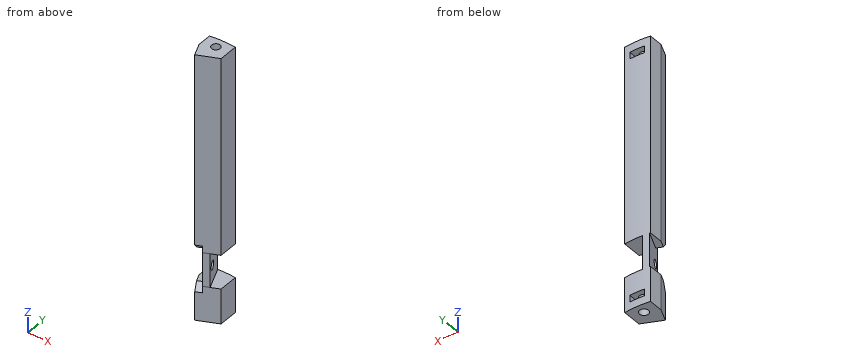
from build123d import *

# Parameters (mm, degrees)
BOSS_EXTRU_2_DEPTH       = 102.5
ESQUISSE8_R              = 1.75
ENL_V_MAT_EXTRU_5_DEPTH  = 11.5
ENL_V_START              = -3
ENL_V_MAT_EXTRU_6_DEPTH  = 2.6
ENL_V_START_2            = -89
ENL_V_MAT_EXTRU_11_DEPTH = 13
ESQUISSE15_R             = 1.625
ENL_V_MAT_EXTRU_12_DEPTH = 109.858621468
CHANFREIN1_SIZE          = 2.5
ESQUISSE16_R             = 1.65
ENL_V_MAT_EXTRU_13_DEPTH = 11.5
ENL_V_START_3            = -5.6
ENL_V_MAT_EXTRU_14_DEPTH = 2.6


with BuildPart() as part:
    # Esquisse3 → Boss.-Extru.2 (new body)
    with BuildSketch(Plane.XY):
        with BuildLine():
            Line((5, 29.665669478), (-2.833530831, 26.427314208))
            Line((-2.833530831, 26.427314208), (-5, 31.657633458))
            Line((-5, 31.657633458), (-5, 37.165171868))
            ThreePointArc((-5, 37.165171868), (0, 37.5), (5, 37.165171868))
            Line((5, 37.165171868), (5, 29.665669478))
        make_face()
    extrude(amount=BOSS_EXTRU_2_DEPTH)

    # Esquisse8 → Enlèv. mat.-Extru.5 (cut)
    with BuildSketch(Plane(origin=(0, 0, 0), x_dir=(-1, 0, 0), z_dir=(0, 0, -1))):
        with Locations((0, 33.75)):
            Circle(ESQUISSE8_R)
    extrude(amount=-ENL_V_MAT_EXTRU_5_DEPTH, mode=Mode.SUBTRACT)

    # Esquisse9 → Enlèv. mat.-Extru.6 (cut)
    with BuildSketch(Plane(origin=(0, 0, 0), x_dir=(-1, 0, 0), z_dir=(0, 0, -1)).offset(ENL_V_START)):
        with BuildLine():
            Line((-2.85, 37.391543162), (-2.85, 31.995448267))
            Line((-2.85, 31.995448267), (0, 30.35))
            Line((0, 30.35), (2.85, 31.995448267))
            Line((2.85, 31.995448267), (2.85, 37.391543162))
            ThreePointArc((2.85, 37.391543162), (0, 37.5), (-2.85, 37.391543162))
        make_face()
    extrude(amount=-ENL_V_MAT_EXTRU_6_DEPTH, mode=Mode.SUBTRACT)

    # Esquisse14 → Enlèv. mat.-Extru.11 (cut)
    with BuildSketch(Plane.XY.offset(102.5).offset(ENL_V_START_2)):
        with BuildLine():
            Line((-2.833530831, 26.427314208), (-0.564385746, 27.365371146))
            Line((-0.564385746, 27.365371146), (-4.642779542, 37.211484761))
            ThreePointArc((-4.642779542, 37.211484761), (-4.821445379, 37.188757232), (-5, 37.165171868))
            Line((-5, 37.165171868), (-5, 31.657633458))
            Line((-5, 31.657633458), (-2.833530831, 26.427314208))
        make_face()
        with BuildLine():
            Line((1.745788964, 28.320930853), (-0.564385746, 27.365371146))
            Line((-0.564385746, 27.365371146), (5, 29.665669478))
            Line((5, 29.665669478), (5, 37.165171868))
            ThreePointArc((5, 37.165171868), (1.48984988, 37.470392943), (-2.03345257, 37.444827021))
            Line((-2.03345257, 37.444827021), (1.745788964, 28.320930853))
        make_face()
    extrude(amount=ENL_V_MAT_EXTRU_11_DEPTH, mode=Mode.SUBTRACT)

    # Esquisse15 → Enlèv. mat.-Extru.12 (cut, through all)
    with BuildSketch(Plane(origin=(11.503085218, 4.764733906, 0), x_dir=(0, 0, -1), z_dir=(0.9238795325112864, 0.38268343236509095, 0))):
        with Locations(Location((-20, 28.49654364, 0), (0, 0, 90))):
            Circle(ESQUISSE15_R)
    extrude(amount=-ENL_V_MAT_EXTRU_12_DEPTH, mode=Mode.SUBTRACT)

    # Chanfrein1
    # the kernel refuses this chamfer: 2.5 mm, written as the material it takes off along each edge
    with BuildSketch(Plane(origin=(-8.775058658, 23.971106609, 13.5), x_dir=(0.010504495520027614, -0.025410210633805018, -0.9996219169112968), z_dir=(0.924146227220892, 0.38203893873974615, 0))) as chanfrein1_piece_1_section:
        Polygon((CHANFREIN1_SIZE * 0.999621916911, CHANFREIN1_SIZE * 0.0274958766106), (-CHANFREIN1_SIZE * 0.0274958766106, CHANFREIN1_SIZE * 0.999621916911), (0, 0), align=None)
    chanfrein1_piece_1 = extrude(amount=8.884603616, mode=Mode.PRIVATE)
    chanfrein1_piece_1 = split(chanfrein1_piece_1, bisect_by=Plane(origin=(-0.88361638, 28.136062073, 12.666666667), z_dir=(-0.9238795325112863, -0.382683432365091, 0)), keep=Keep.TOP, mode=Mode.PRIVATE)
    add(chanfrein1_piece_1, mode=Mode.SUBTRACT)
    with BuildSketch(Plane(origin=(-8.775058658, 23.971106609, 26.5), x_dir=(-0.38189449627778244, 0.9237968231608907, -0.027495876610586317), z_dir=(0.924146227220892, 0.38203893873974615, 0))) as chanfrein1_piece_2_section:
        Polygon((CHANFREIN1_SIZE * 0.999621916911, CHANFREIN1_SIZE * 0.0274958766106), (-CHANFREIN1_SIZE * 0.0274958766106, CHANFREIN1_SIZE * 0.999621916911), (0, 0), align=None)
    chanfrein1_piece_2 = extrude(amount=8.884603616, mode=Mode.PRIVATE)
    chanfrein1_piece_2 = split(chanfrein1_piece_2, bisect_by=Plane(origin=(-0.88361638, 28.136062073, 27.333333333), z_dir=(-0.9238795325112863, -0.382683432365091, 0)), keep=Keep.TOP, mode=Mode.PRIVATE)
    add(chanfrein1_piece_2, mode=Mode.SUBTRACT)

    # Esquisse16 → Enlèv. mat.-Extru.13 (cut)
    with BuildSketch(Plane.XY.offset(102.5)):
        with Locations((0, 33.75)):
            Circle(ESQUISSE16_R)
    extrude(amount=-ENL_V_MAT_EXTRU_13_DEPTH, mode=Mode.SUBTRACT)

    # Esquisse17 → Enlèv. mat.-Extru.14 (cut)
    with BuildSketch(Plane.XY.offset(102.5).offset(ENL_V_START_3)):
        with BuildLine():
            Line((-2.85, 37.391543162), (-2.85, 31.995448267))
            Line((-2.85, 31.995448267), (0, 30.35))
            Line((0, 30.35), (2.85, 31.995448267))
            Line((2.85, 31.995448267), (2.85, 37.391543162))
            ThreePointArc((2.85, 37.391543162), (0, 37.5), (-2.85, 37.391543162))
        make_face()
    extrude(amount=ENL_V_MAT_EXTRU_14_DEPTH, mode=Mode.SUBTRACT)


solid = part.part
Check sheet for the modelled part. Datum: model origin and axes. Units: mm. Round coordinates to 2 decimals unless told otherwise and drop trailing zeros. Loops run counter-clockwise (first coordinate to the right, second up) from the corner with the lowest first, then second, coordinate; pieces in that order, holes last. Notation, with made-up numbers: M 62.5,-15.75 L 72.5,-15.75 A16 ccw 72.5,-11.75 Z; hole C -12,5 d8. An arc over 180 degrees is marked long. One line per item, written item: value.
(1) Thickness scan on line 1 (Z direction, x = 2.25, y = 33.5); line 2 (Z direction, x = -0.25, y = 30.75); line 3 (Z direction, x = -3.25, y = 29.25). Record the ranges inside material, lowest first.
Computed values:
line 1: z = 0 to 3, 5.6 to 13.5, 26.5 to 96.9, 99.5 to 102.5
line 2: z = 0 to 3, 5.6 to 18.38, 21.62 to 96.9, 99.5 to 102.5
line 3: z = 0 to 13.5, 26.5 to 102.5
(2) Depth check by flat-ended pin: pin 1 Ø2.5 at (x, y) = (0, 33.75) entering from -Z; pin 2 Ø2 at (x, y) = (0, 33.75) entering from +Z; pin 3 Ø1.5 at (x, z) = (3.5, 47) entering from +Y. Enter the tip coordinate at first touch or a pass-through.
Computed values:
pin 1: stops at z = 11.5
pin 2: stops at z = 91
pin 3: stops at y = 37.4
(3) Sectioned sample at B-B, the plane z = 85.5. Record the cut outline in (x, y).
Computed values:
outline: M -5,31.66 L -2.83,26.43 L 5,29.67 L 5,37.17 A37.5 ccw -5,37.17 Z
(4) Sectioned sample at A-A, the plane z = 9. Record the cut outline in (x, y).
Computed values:
outline: M -5,31.66 L -2.83,26.43 L 5,29.67 L 5,37.17 A37.5 ccw -5,37.17 Z; hole C 0,33.75 d3.5
